from build123d import *

# Parameters (mm, degrees)
BOSS_EXTRUDE1_DEPTH  = 3.81
SKETCH2_W            = 30.48
SKETCH2_H            = 48.26
CUT_EXTRUDE1_DEPTH   = 3.81
SKETCH4_W            = 30.48
SKETCH4_H            = 3.81
CUT_EXTRUDE2_DEPTH   = 27.94
SKETCH5_W            = 0.25
SKETCH5_H            = 3.81
CUT_EXTRUDE3_DEPTH   = 53.07
CUT_EXTRUDE4_DEPTH   = 7.874
BOSS_EXTRUDE2_DEPTH  = 1.27
SKETCH8_R            = 1.524
CUT_EXTRUDE6_DEPTH   = 6.08
SKETCH9_W            = 5.08
SKETCH9_H            = 5.08
CUT_EXTRUDE7_DEPTH   = 70.883682204
SKETCH10_OUTSIDE_W   = 96.904
SKETCH10_OUTSIDE_H   = 92.332
SKETCH10_OUTSIDE_W_2 = 56.38
SKETCH10_OUTSIDE_H_2 = 76.267364408
CUT_EXTRUDE8_DEPTH   = 6.08
SKETCH11_W           = 26.4
SKETCH11_H           = 2.57
SKETCH11_W_2         = 2.57
SKETCH11_H_2         = 26.4
BOSS_EXTRUDE4_DEPTH  = 4.62
SKETCH12_R           = 5.92
CUT_EXTRUDE9_DEPTH   = 57.38
SKETCH13_R           = 5.92
CUT_EXTRUDE10_DEPTH  = 70.883682204


with BuildPart() as part:
    # Sketch1 → Boss-Extrude1 (new body)
    with BuildSketch(Plane.XZ.offset(12.45)):
        Polygon((-12.7, 31.75), (12.7, 31.75), (27.068409794, 17.381590206), (37.228409794, -0.216045999), (37.228409794, -20.536045999), (27.068409794, -38.133682204), (-27.068409794, -38.133682204), (-37.228409794, -20.536045999), (-37.228409794, -0.216045999), (-27.068409794, 17.381590206), align=None)
    extrude(amount=-BOSS_EXTRUDE1_DEPTH)

    # Sketch2 → Cut-Extrude1 (cut)
    with BuildSketch(Plane.XZ.offset(12.45)):
        with Locations((0, 1.27)):
            Rectangle(SKETCH2_W, SKETCH2_H)
    extrude(amount=-CUT_EXTRUDE1_DEPTH, mode=Mode.SUBTRACT)

    # Sketch4 → Cut-Extrude2 (cut)
    with BuildSketch(Plane(origin=(0, 0, 25.4), x_dir=(-1, 0, 0), z_dir=(0, 0, -1))):
        with Locations((0, -10.545)):
            Rectangle(SKETCH4_W, SKETCH4_H)
    extrude(amount=-CUT_EXTRUDE2_DEPTH, mode=Mode.SUBTRACT)

    # Sketch5 → Cut-Extrude3 (cut, through all)
    with BuildSketch(Plane.XY.offset(-22.86)):
        with Locations((-15.365, -10.545)):
            Rectangle(SKETCH5_W, SKETCH5_H)
        with Locations((15.365, -10.545)):
            Rectangle(SKETCH5_W, SKETCH5_H)
    extrude(amount=CUT_EXTRUDE3_DEPTH, mode=Mode.SUBTRACT)

    # Sketch6 → Cut-Extrude4 (cut)
    with BuildSketch(Plane.XY.offset(-22.86)):
        Polygon((7.62, -12.45), (15.24, -12.45), (15.24, -9.275), (11.557, -9.275), (7.62, -9.275), align=None)
        Polygon((-15.24, -12.45), (-15.24, -9.275), (-11.557, -9.275), (-7.62, -9.275), (-7.62, -12.45), align=None)
    extrude(amount=-CUT_EXTRUDE4_DEPTH, mode=Mode.SUBTRACT)

    # Sketch1_3 → Boss-Extrude2 (add)
    with BuildSketch(Plane.XZ.offset(12.45)):
        Polygon((-12.7, 31.75), (12.7, 31.75), (27.068409794, 17.381590206), (37.228409794, -0.216045999), (37.228409794, -20.536045999), (27.068409794, -38.133682204), (-27.068409794, -38.133682204), (-37.228409794, -20.536045999), (-37.228409794, -0.216045999), (-27.068409794, 17.381590206), align=None)
    extrude(amount=BOSS_EXTRUDE2_DEPTH)

    # Sketch8 → Cut-Extrude6 (cut, through all)
    with BuildSketch(Plane.XZ.offset(13.72)):
        with Locations((-8.89, 22.86)):
            Circle(SKETCH8_R)
        with Locations((8.89, 22.86)):
            Circle(SKETCH8_R)
    extrude(amount=-CUT_EXTRUDE6_DEPTH, mode=Mode.SUBTRACT)

    # Sketch9 → Cut-Extrude7 (cut, through all)
    with BuildSketch(Plane(origin=(0, 0, -38.133682204), x_dir=(-1, 0, 0), z_dir=(0, 0, -1))):
        with Locations((0.7493, -8.5252)):
            Rectangle(SKETCH9_W, SKETCH9_H)
    extrude(amount=-CUT_EXTRUDE7_DEPTH, mode=Mode.SUBTRACT)

    # Sketch10 outside → Cut-Extrude8 (cut, through all)
    with BuildSketch(Plane.XZ.offset(13.72)):
        with Locations((0, -3.192)):
            Rectangle(SKETCH10_OUTSIDE_W, SKETCH10_OUTSIDE_H)
        Rectangle(SKETCH10_OUTSIDE_W_2, SKETCH10_OUTSIDE_H_2, mode=Mode.SUBTRACT)
    extrude(amount=-CUT_EXTRUDE8_DEPTH, mode=Mode.SUBTRACT)

    # Sketch11 → Boss-Extrude4 (add)
    with BuildSketch(Plane.XZ.offset(13.72)):
        with BuildLine():
            Line((22.725, 21.725), (12.7, 31.75))
            Line((12.7, 31.75), (-12.7, 31.75))
            Line((-12.7, 31.75), (-22.725, 21.725))
            Line((-22.725, 21.725), (-9.907030481, 21.725))
            ThreePointArc((-9.907030481, 21.725), (-9.511539036, 24.251497476), (-7.366, 22.86))
            ThreePointArc((-7.366, 22.86), (-7.498502524, 22.238460964), (-7.872969519, 21.725))
            Line((-7.872969519, 21.725), (7.872969519, 21.725))
            ThreePointArc((7.872969519, 21.725), (8.268460964, 24.251497476), (10.414, 22.86))
            ThreePointArc((10.414, 22.86), (10.281497476, 22.238460964), (9.907030481, 21.725))
            Line((9.907030481, 21.725), (22.725, 21.725))
        make_face()
        with Locations((0, 26.185)):
            Rectangle(SKETCH11_W, SKETCH11_H, mode=Mode.SUBTRACT)
        Polygon((-27.068409794, -38.133682204), (-18.165, -38.133682204), (-18.165, 3.641317796), (-28.19, 3.641317796), (-28.19, -36.191030981), align=None)
        with Locations((-22.625, -12.733682204)):
            Rectangle(SKETCH11_W_2, SKETCH11_H_2, mode=Mode.SUBTRACT)
        Polygon((28.19, -36.191030981), (28.19, 3.641317796), (18.165, 3.641317796), (18.165, -38.133682204), (27.068409794, -38.133682204), align=None)
        with Locations((22.625, -12.733682204)):
            Rectangle(SKETCH11_W_2, SKETCH11_H_2, mode=Mode.SUBTRACT)
    extrude(amount=BOSS_EXTRUDE4_DEPTH)

    # Sketch12 → Cut-Extrude9 (cut, through all)
    with BuildSketch(Plane(origin=(28.19, 0, 0), x_dir=(0, 0, -1), z_dir=(1, 0, 0))):
        with Locations((12.735281649, -22.602468851)):
            Circle(SKETCH12_R)
    extrude(amount=-CUT_EXTRUDE9_DEPTH, mode=Mode.SUBTRACT)

    # Sketch13 → Cut-Extrude10 (cut, through all)
    with BuildSketch(Plane.XY.offset(31.75)):
        with Locations((-0.001599445, -22.617531149)):
            Circle(SKETCH13_R)
    extrude(amount=-CUT_EXTRUDE10_DEPTH, mode=Mode.SUBTRACT)


solid = part.part
Input: part model. Units: mm. Frame: model coordinates. A direction names the side the tool comes from. Round coordinates to 2 decimals unless told otherwise and drop trailing zeros. Write each loop counter-clockwise with the first axis right and the second up, starting at its lowest first coordinate (ties: lowest second). Pieces come first, ordered by that corner, then holes.
1) Cut plane D-D (x = -20). Return the cut outline in (y, z) (3 decimals).
2) Cut plane B-B (x = -8.89). Return the cut outline in (y, z) (3 decimals).
3) Ray query, L1, parallel to X at y = -15.5, z = -7.5 (3 decimals); L2, parallel to Z at x = 8.89, y = -17.1; L3, parallel to Z at x = -4, y = -17.5 (3 decimals). Return the intervals inside material, ascending.
4) Cut plane A-A (y = -10). Return the cut outline in (x, z), then the cut area to 3 significant figures.
5) Draft query along Z for faces 4 (the flat face through (-3.289, -10, -31)), 5 (the flat face through (-23.91, -16, -13)), 6 (the flat face through (0, -16, 21.725)), 7 (the flat face through (19.98, -13.42, 24.47)). Return one class per face: pulls with the +Z half, pulls with the -Z half, needs draft (parallel to the pull), parting line crosses it, or undercut.
6) Reachability of faces 1 (the flat face through (0, -16, 27.47)), 2 (the flat face through (11, -9.275, -27)), 3 (the flat face through (23, -18.34, -27)) from +Z, -Z, +X, -X, +Y, -Y: full face, straight path, thin tool, end or side. Return the list, or none.
7) Contact query for flat-ended pins moving along their axis: P1, Ø12, axis at x = -0.5, z = -7.5, coming from the -Y side; P2, Ø4, axis at x = 8.89, z = 22.86, coming from the +Y side; P3, Ø1, axis at x = 20, y = -11, coming from the +Z side. Output: stop coordinate, or through.
8) Cut plane C-C (z = 6.5). Return the cut outline in (x, y).
Geometry says:
1. outline: (-18.34, -38.134) - (-8.64, -38.134) - (-8.64, 24.45) - (-18.34, 24.45) - (-18.34, 21.725) - (-13.72, 21.725) - (-13.72, 3.641) - (-18.34, 3.641) - (-18.34, -8.627) arc R5.92 cw to (-18.34, -16.844) - close
2. outline: (-18.34, 24.384) - (-12.45, 24.384) - (-12.45, 31.75) - (-18.34, 31.75) - (-18.34, 27.47) - (-13.72, 27.47) - (-13.72, 24.9) - (-18.34, 24.9) - close; (-13.72, -38.134) - (-8.64, -38.134) - (-8.64, -22.86) - (-9.275, -22.86) - (-9.275, -30.734) - (-12.45, -30.734) - (-12.45, 21.336) - (-13.72, 21.336) - close
3. L1: x = -28.19 to -23.91, -21.34 to -18.165, 18.165 to 21.34, 23.91 to 28.19
3. L2: z = 24.38 to 24.9, 27.47 to 31.75
3. L3: z = 21.725 to 24.9, 27.47 to 31.75
4. outline: (-28.19, -36.19) - (-27.07, -38.13) - (-3.29, -38.13) - (-3.29, -22.86) - (-7.62, -22.86) - (-7.62, -30.73) - (-15.24, -30.73) - (-15.24, -22.86) - (-15.49, -22.86) - (-15.49, 28.96) - (-27.07, 17.38) - (-28.19, 15.44) - close; (1.79, -38.13) - (27.07, -38.13) - (28.19, -36.19) - (28.19, 15.44) - (27.07, 17.38) - (15.49, 28.96) - (15.49, -22.86) - (15.24, -22.86) - (15.24, -30.73) - (7.62, -30.73) - (7.62, -22.86) - (1.79, -22.86) - close
4. area: 1,820 mm2
5. face 4: needs draft
5. face 5: undercut
5. face 6: pulls with the -Z half
5. face 7: pulls with the +Z half
6. face 1: -Y
6. face 2: +Z
6. face 3: +Z, -Z, +X, -X, -Y
7. P1: stops at y = -13.72
7. P2: stops at y = -12.45
7. P3: stops at z = 24.95
8. outline: (-28.19, -13.72) - (28.19, -13.72) - (28.19, -8.64) - (15.49, -8.64) - (15.49, -12.45) - (-15.49, -12.45) - (-15.49, -8.64) - (-28.19, -8.64) - close
